For this review, take the finished solid that the model builds, in its own axes (mm). A direction names the side the tool comes from. Round coordinates to 2 decimals unless told otherwise and drop trailing zeros. Write each loop counter-clockwise with the first axis right and the second up, starting at its lowest first coordinate (ties: lowest second). Pieces come first, ordered by that corner, then holes. Notation, with made-up numbers: M 87.25,15 L 145.25,15 A14 cw 145.25,37 Z; hole C -1.75,34.25 d3. An arc over 180 degrees is marked long. Answer in a Markdown table with one row per item.
```python
from build123d import *

# Parameters (mm, degrees)
EXTRUDE_1_DEPTH                 = 20
CUT_EXTRUDE_1_REACH             = 60.241
SKETCH_2_R                      = 4
CUT_EXTRUDE_1_DIRECTION_2_DEPTH = 59.241379608
CUT_EXTRUDE_2_REACH             = 60.241
SKETCH_3_R                      = 1.4
SKETCH_3_R_2                    = 1
SKETCH_7_W                      = 10
SKETCH_7_H                      = 32.195121952
EXTRUDE_2_DEPTH                 = 2
SKETCH_8_W                      = 43
SKETCH_8_H                      = 10
EXTRUDE_3_DEPTH                 = 2
SKETCH_9_W                      = 10
SKETCH_9_H                      = 30.195121952
EXTRUDE_4_DEPTH                 = 2
SKETCH_11_R                     = 1.4
SKETCH_11_R_2                   = 4
CUT_EXTRUDE_8_DEPTH             = 2
SKETCH_13_W                     = 45
SKETCH_13_H                     = 5
EXTRUDE_5_DEPTH                 = 2
SKETCH_14_W                     = 2
SKETCH_14_H                     = 5
EXTRUDE_6_DEPTH                 = 30.19512195
CUT_EXTRUDE_9_REACH             = 48.559
SKETCH_19_R                     = 1.5
SKETCH_19_R_2                   = 3


with BuildPart() as part:
    # 草图1 → 凸台-拉伸1 (new body)
    with BuildSketch(Plane.XY):
        Polygon((22.5, 1.097560976), (22.5, -1.097560976), (-22.5, -1.097560976), (-22.5, 1.097560976), (-22.5, 31.097560976), (-20.5, 31.097560976), (-20.5, 0.902439024), (20.5, 0.902439024), (20.5, 31.097560976), (22.5, 31.097560976), align=None)
    extrude(amount=EXTRUDE_1_DEPTH)

    # 草图2 → 切除-拉伸1 (cut, up to next)
    with BuildSketch(Plane.ZY.offset(22.5), mode=Mode.PRIVATE) as cut_extrude_1_sk1:
        with Locations(Location((10, 14.146341463, 0), (0, 0, 90))):
            Circle(SKETCH_2_R)
    cut_extrude_1_tool1 = extrude(cut_extrude_1_sk1.sketch, amount=-CUT_EXTRUDE_1_REACH, mode=Mode.PRIVATE) & part.part
    add(cut_extrude_1_tool1.solids().sort_by_distance((-22.5, 14.146341, 10))[0], mode=Mode.SUBTRACT)

    # 草图2 → 切除-拉伸1 direction 2 (cut)
    with BuildSketch(Plane.ZY.offset(22.5)):
        with Locations(Location((10, 14.146341463, 0), (0, 0, 90))):
            Circle(SKETCH_2_R)
    extrude(amount=CUT_EXTRUDE_1_DIRECTION_2_DEPTH, mode=Mode.SUBTRACT)

    # 草图3 → 切除-拉伸2 (cut, up to next)
    with BuildSketch(Plane.ZY.offset(22.5), mode=Mode.PRIVATE) as cut_extrude_2_sk1:
        with Locations(Location((2, 22.096341464, 0), (0, 0, 270))):
            Circle(SKETCH_3_R)
    cut_extrude_2_tool1 = extrude(cut_extrude_2_sk1.sketch, amount=-CUT_EXTRUDE_2_REACH, mode=Mode.PRIVATE) & part.part
    # 草图3 → 切除-拉伸2 (cut, up to next)
    with BuildSketch(Plane.ZY.offset(22.5), mode=Mode.PRIVATE) as cut_extrude_2_sk2:
        with Locations(Location((18, 22.12195122, 0), (0, 0, 270))):
            Circle(SKETCH_3_R_2)
    cut_extrude_2_tool2 = extrude(cut_extrude_2_sk2.sketch, amount=-CUT_EXTRUDE_2_REACH, mode=Mode.PRIVATE) & part.part
    # 草图3 → 切除-拉伸2 (cut, up to next)
    with BuildSketch(Plane.ZY.offset(22.5), mode=Mode.PRIVATE) as cut_extrude_2_sk3:
        with Locations((18, 6.12195122)):
            Circle(SKETCH_3_R_2)
    cut_extrude_2_tool3 = extrude(cut_extrude_2_sk3.sketch, amount=-CUT_EXTRUDE_2_REACH, mode=Mode.PRIVATE) & part.part
    # 草图3 → 切除-拉伸2 (cut, up to next)
    with BuildSketch(Plane.ZY.offset(22.5), mode=Mode.PRIVATE) as cut_extrude_2_sk4:
        with Locations((2, 6.171951224)):
            Circle(SKETCH_3_R)
    cut_extrude_2_tool4 = extrude(cut_extrude_2_sk4.sketch, amount=-CUT_EXTRUDE_2_REACH, mode=Mode.PRIVATE) & part.part
    add(cut_extrude_2_tool1.solids().sort_by_distance((-22.5, 22.096341, 2))[0], mode=Mode.SUBTRACT)
    add(cut_extrude_2_tool2.solids().sort_by_distance((-22.5, 22.121951, 18))[0], mode=Mode.SUBTRACT)
    add(cut_extrude_2_tool3.solids().sort_by_distance((-22.5, 6.121951, 18))[0], mode=Mode.SUBTRACT)
    add(cut_extrude_2_tool4.solids().sort_by_distance((-22.5, 6.171951, 2))[0], mode=Mode.SUBTRACT)

    # 草图7 → 凸台-拉伸2 (add)
    with BuildSketch(Plane(origin=(22.5, 0, 0), x_dir=(0, 0, -1), z_dir=(1, 0, 0))):
        with Locations((5, 15)):
            Rectangle(SKETCH_7_W, SKETCH_7_H)
    extrude(amount=-EXTRUDE_2_DEPTH)

    # 草图8 → 凸台-拉伸3 (add)
    with BuildSketch(Plane.XZ.offset(1.097560976)):
        with Locations((-1, -5)):
            Rectangle(SKETCH_8_W, SKETCH_8_H)
    extrude(amount=-EXTRUDE_3_DEPTH)

    # 草图9 → 凸台-拉伸4 (add)
    with BuildSketch(Plane.ZY.offset(22.5)):
        with Locations((-5, 16)):
            Rectangle(SKETCH_9_W, SKETCH_9_H)
    extrude(amount=-EXTRUDE_4_DEPTH)

    # 草图11 → 切除-拉伸8 (cut)
    with BuildSketch(Plane(origin=(22.5, 0, 0), x_dir=(0, 0, -1), z_dir=(1, 0, 0))):
        with Locations(Location((4, 20.741461029, 0), (0, 0, 90))):
            Circle(SKETCH_11_R)
        with Locations(Location((4, 6.741461029, 0), (0, 0, 90))):
            Circle(SKETCH_11_R)
        with Locations(Location((-3, 13.741461029, 0), (0, 0, 90))):
            Circle(SKETCH_11_R)
        with Locations(Location((4, 13.741461029, 0), (0, 0, 90))):
            Circle(SKETCH_11_R_2)
    extrude(amount=-CUT_EXTRUDE_8_DEPTH, mode=Mode.SUBTRACT)

    # 草图13 → 凸台-拉伸5 (add)
    with BuildSketch(Plane.XZ.offset(1.097560976)):
        with Locations((0, 22.5)):
            Rectangle(SKETCH_13_W, SKETCH_13_H)
    extrude(amount=-EXTRUDE_5_DEPTH)

    # 草图14 → 凸台-拉伸6 (add)
    with BuildSketch(Plane(origin=(0, 0.902439024, 0), x_dir=(1, 0, 0), z_dir=(0, 1, 0))):
        with Locations((21.5, -22.5)):
            Rectangle(SKETCH_14_W, SKETCH_14_H)
        with Locations((-21.5, -22.5)):
            Rectangle(SKETCH_14_W, SKETCH_14_H)
    extrude(amount=EXTRUDE_6_DEPTH)

    # 草图19 → 切除-拉伸9 (cut, up to next)
    with BuildSketch(Plane.XZ.offset(1.097560976), mode=Mode.PRIVATE) as cut_extrude_9_sk1:
        with Locations((-5, 20)):
            Circle(SKETCH_19_R)
    cut_extrude_9_tool1 = extrude(cut_extrude_9_sk1.sketch, amount=-CUT_EXTRUDE_9_REACH, mode=Mode.PRIVATE) & part.part
    # 草图19 → 切除-拉伸9 (cut, up to next)
    with BuildSketch(Plane.XZ.offset(1.097560976), mode=Mode.PRIVATE) as cut_extrude_9_sk2:
        with Locations((0, 15)):
            Circle(SKETCH_19_R_2)
    cut_extrude_9_tool2 = extrude(cut_extrude_9_sk2.sketch, amount=-CUT_EXTRUDE_9_REACH, mode=Mode.PRIVATE) & part.part
    # 草图19 → 切除-拉伸9 (cut, up to next)
    with BuildSketch(Plane.XZ.offset(1.097560976), mode=Mode.PRIVATE) as cut_extrude_9_sk3:
        with Locations(Location((-5, 10, 0), (0, 0, 270))):
            Circle(SKETCH_19_R)
    cut_extrude_9_tool3 = extrude(cut_extrude_9_sk3.sketch, amount=-CUT_EXTRUDE_9_REACH, mode=Mode.PRIVATE) & part.part
    # 草图19 → 切除-拉伸9 (cut, up to next)
    with BuildSketch(Plane.XZ.offset(1.097560976), mode=Mode.PRIVATE) as cut_extrude_9_sk4:
        with Locations((5, 10)):
            Circle(SKETCH_19_R)
    cut_extrude_9_tool4 = extrude(cut_extrude_9_sk4.sketch, amount=-CUT_EXTRUDE_9_REACH, mode=Mode.PRIVATE) & part.part
    # 草图19 → 切除-拉伸9 (cut, up to next)
    with BuildSketch(Plane.XZ.offset(1.097560976), mode=Mode.PRIVATE) as cut_extrude_9_sk5:
        with Locations(Location((5, 20, 0), (0, 0, 270))):
            Circle(SKETCH_19_R)
    cut_extrude_9_tool5 = extrude(cut_extrude_9_sk5.sketch, amount=-CUT_EXTRUDE_9_REACH, mode=Mode.PRIVATE) & part.part
    add(cut_extrude_9_tool1.solids().sort_by_distance((-5, -1.097561, 20))[0], mode=Mode.SUBTRACT)
    add(cut_extrude_9_tool2.solids().sort_by_distance((0, -1.097561, 15))[0], mode=Mode.SUBTRACT)
    add(cut_extrude_9_tool3.solids().sort_by_distance((-5, -1.097561, 10))[0], mode=Mode.SUBTRACT)
    add(cut_extrude_9_tool4.solids().sort_by_distance((5, -1.097561, 10))[0], mode=Mode.SUBTRACT)
    add(cut_extrude_9_tool5.solids().sort_by_distance((5, -1.097561, 20))[0], mode=Mode.SUBTRACT)


solid = part.part
```
Q1. For probe 1 along X at (y, z) = (28.5, 1.5); probe 2 along Y at (x, z) = (-21, 10); probe 3 along Y at (x, z) = (1.5, -3), list the stretches that pass through material, from the lowest coordinate up.
Found:
| item | result |
|---|---|
| probe 1 | -22.5 to -20.5, 20.5 to 22.5 |
| probe 2 | -1.1 to 10.15, 18.15 to 31.1 |
| probe 3 | -1.1 to 0.9 |
Q2. Insertion check: P1, Ø1.2, axis at y = 6.12, z = 18, coming from the -X side; P2, Ø2.5, axis at x = 5, z = 10, coming from the +Y side; P3, Ø7, axis at y = 13.74, z = -4, coming from the +X side; P4, Ø17.5, axis at x = -9, z = -1, coming from the +Y side. Each pin has a flat end and moves straight along its axis. Give the tip position at first contact, or say it passes through.
Found:
| item | result |
|---|---|
| P1 | x = 20.5 |
| P2 | through |
| P3 | x = -20.5 |
| P4 | y = 0.9 |
Q3. Take a section at B-B (z = 15). State the section outline as (x, y) points.
Found:
| item | result |
|---|---|
| outline | M -22.5,-1.1 L -3,-1.1 L -3,0.9 L -20.5,0.9 L -20.5,31.1 L -22.5,31.1 Z; M 3,-1.1 L 22.5,-1.1 L 22.5,31.1 L 20.5,31.1 L 20.5,0.9 L 3,0.9 Z |
Q4. Take a section at D-D (x = -5). State the section outline as (y, z) points.
Found:
| item | result |
|---|---|
| outline | M -1.1,-10 L 0.9,-10 L 0.9,8.5 L -1.1,8.5 Z; M -1.1,11.5 L 0.9,11.5 L 0.9,18.5 L -1.1,18.5 Z; M -1.1,21.5 L 0.9,21.5 L 0.9,25 L -1.1,25 Z |
Q5. Mouldability with a two-part tool opening along X and no side actions: class faces 6 (the face through (-21.51, 5.32, 0.89)), 7 (the face through (-22.5, 11, 7)), 8 (the face through (20.5, 16, 8)) as +X half, -X half, draft (parallel to the pull), parting line (faces both ways), or undercut.
Found:
| item | result |
|---|---|
| face 6 | draft |
| face 7 | -X half |
| face 8 | undercut |
Q6. Take a section at A-A (x = 0). State the section outline as (y, z) points.
Found:
| item | result |
|---|---|
| outline | M -1.1,-10 L 0.9,-10 L 0.9,12 L -1.1,12 Z; M -1.1,18 L 0.9,18 L 0.9,25 L -1.1,25 Z |
Q7. Take a section at C-C (z = 20). State the section outline as (x, y) points.
Found:
| item | result |
|---|---|
| outline | M -22.5,-1.1 L -6.5,-1.1 L -6.5,0.9 L -20.5,0.9 L -20.5,31.1 L -22.5,31.1 Z; M -3.5,-1.1 L 3.5,-1.1 L 3.5,0.9 L -3.5,0.9 Z; M 6.5,-1.1 L 22.5,-1.1 L 22.5,31.1 L 20.5,31.1 L 20.5,0.9 L 6.5,0.9 Z |
Q8. Machinability: for faces 1 (the face through (21.514, 22.035, -4.536)), 2 (the face through (0, 0.902, 8)), 3 (the face through (-21.514, 22.4, 0.633)), 4 (the face through (0, -1.098, 8)), 5 (the face through (5.07, -0.11, 21.5)), which of the approach directions +Z, -Z, +X, -X, +Y, -Y give a long, thin tool a straight path to every point of the face, cutting with its end or side? Answer none if there is none.
Found:
| item | result |
|---|---|
| face 1 | +X |
| face 2 | +Z, -Z, +Y |
| face 3 | -X |
| face 4 | +Z, -Z, +X, -X, -Y |
| face 5 | +Y, -Y |
